Source: CAD feature listing. Evaluate the final solid. Frame: model axes, mm. Face numbers are marked on the shaded views. A direction names the side the tool comes from. Coordinates: 2 decimals unless noted, no trailing zeros. Write each loop counter-clockwise with the first axis right and the second up, starting at its lowest first coordinate (ties: lowest second). Pieces come first, ordered by that corner, then holes. Notation, with made-up numbers: M 87,-34.5 L 143,-34.5 A9 ccw 143,-23.5 Z; hole C -23,58 d3. An arc over 180 degrees is marked long. One line per item, written item: value. Start each with the question number.
Item 1: Pin query (flat end, axial travel): P1, Ø5, axis at x = 15, y = 13, coming from the -Z side; P2, Ø9.5, axis at x = 18.5, y = 10.5, coming from the +Z side; P3, Ø5, axis at y = 7, z = 20.5, coming from the -X side. Return the tip coordinate at first contact, or that it passes through.
Item 2: Ray query, L1, parallel to X at y = 10.25, z = 25.5; L2, parallel to Z at x = -1, y = 4; L3, parallel to Z at x = 43.5, y = 6. Return the intervals inside material, ascending. Write a range as from..to.
Item 3: Cut plane D-D, the plane z = 10. Output: boundary loops of the cut face in (x, y), then the cut area to 3 significant figures.
Item 4: Set-up query: the marked faces 1, 2, 3 and 4. Return all of +Z, -Z, +X, -X, +Y, -Y with unobstructed straight access to the full face (end or side cutting, diameter ignored); none if empty.
Item 5: Mould query, pull axis X, two halves, no side actions, for the marked faces 5, 6 and 7. Classes: released by +X, released by -X, zero draft, split by the parting line, or undercut.
Item 6: Cut plane A-A, the plane z = 18. Output: boundary loops of the cut face in (x, y), then the cut area to 3 significant figures.
Item 7: Cut plane C-C, the plane x = 26.5. Output: boundary loops of the cut face in (y, z), then the cut area to 3 significant figures.
Item 8: Cut plane B-B, the plane y = 8.75. Output: boundary loops of the cut face in (x, z).
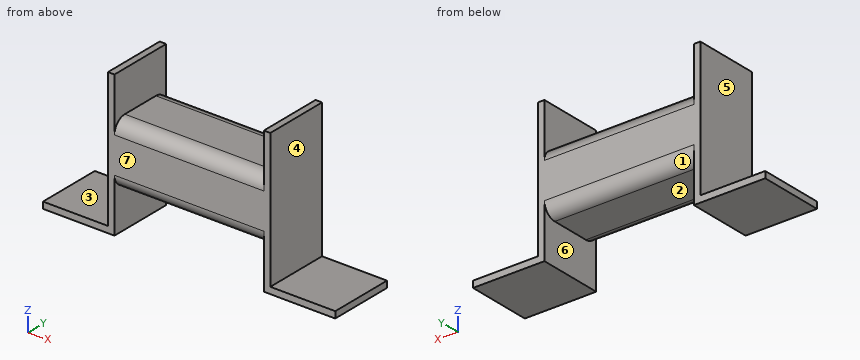
Autodesk Fusion 360 part; units mm, degrees
sketch "Sketch1" plane through (0, 0, 0) normal (0, 1, 0) x (1, 0, 0)
  line L0 (50, 0) -> (50, -15)
  line L1 (0, -15) -> (0, 0)
  line L2 (50, -15) -> (50, -27.5)
  line L3 (50, -27.5) -> (70, -27.5)
  line L4 (70, -27.5) -> (70, -29.5)
  line L5 (70, -29.5) -> (50, -29.5)
  line L6 (50, -29.5) -> (48, -29.5)
  line L7 (48, -29.5) -> (48, -17)
  line L8 (48, -17) -> (2, -17)
  line L9 (2, -17) -> (2, -29.5)
  line L10 (2, -29.5) -> (-20, -29.5)
  line L11 (-20, 14.5) -> (2, 14.5)
  line L12 (2, 14.5) -> (2, 2)
  line L13 (2, 2) -> (48, 2)
  line L14 (48, 2) -> (48, 14.5)
  line L15 (48, 14.5) -> (70, 14.5)
  line L16 (70, 14.5) -> (70, 12.5)
  line L17 (70, 12.5) -> (50, 12.5)
  line L18 (50, 12.5) -> (50, 0)
  line L19 (-20, 14.5) -> (-20, 12.5)
  line L20 (-20, 12.5) -> (0, 12.5)
  line L21 (0, 12.5) -> (0, 0)
  line L22 (-20, -29.5) -> (-20, -27.5)
  line L23 (-20, -27.5) -> (0, -27.5)
  line L24 (0, -27.5) -> (0, -15)
  dimension "d1" = 50
  dimension "d2" = 15
  dimension "d3" = 12.5
  dimension "d4" = 20
  dimension "d5" = 2
  dimension "d6" = 20
  dimension "d7" = 2
  dimension "d8" = 12.5
  dimension "d9" = 46
  dimension "d10" = 12.5
  dimension "d11" = 22
  dimension "d12" = 44
  dimension "d13" = 22
  dimension "d14" = 12.5
  dimension "d15" = 46
  dimension "d16" = 12.5
  dimension "d17" = 22
  dimension "d18" = 2
  dimension "d19" = 20
  dimension "d20" = 2
  dimension "d21" = 20
  dimension "d23" = 2
extrude "Extrude1" add sketch "Sketch1" along normal blind 20
fillet "Fillet1" radius 4 1 edges at (25, 20, 17)
fillet "Fillet2" radius 4 1 edges at (25, 0, 17)
fillet "Fillet3" radius 4 1 edges at (25, 20, -2)
fillet "Fillet4" radius 4 1 edges at (25, 0, -2)
sketch "Sketch2" plane through (50, 0, 0) normal (1, 0, 0) x (0, 0, -1)
  line L0 (-27.5, 0) -> (12.5, 0)
  line L1 (12.5, 0) -> (12.5, 20)
  line L2 (12.5, 20) -> (-27.5, 20)
  line L3 (-27.5, 20) -> (-27.5, 0)
extrude "Extrude2" cut 1 faces at (70, 6.6667, 28.1667) along direction (-1, 0, 0) blind 20
extrude "Extrude3" cut 1 faces at (-20, 6.6667, 28.8333) along direction (1, 0, 0) blind 20
From the geometry:
1. P1: stops at z = -2
1. P2: stops at z = 17
1. P3: stops at x = 0
2. L1: x = 0..2, 48..50
2. L2: z = -14.5..-12.5
2. L3: z = -2..17
3. outline: M 0,0 L 50,0 L 50,20 L 0,20 Z
3. area: 1,000 mm²
4. face 1: -Z, +Y
4. face 2: -Z, +Y, -Y
4. face 3: +Z, -X, +Y, -Y
4. face 4: +Z, +X, +Y, -Y
5. face 5: released by -X
5. face 6: undercut
5. face 7: zero draft
6. outline: M 0,0 L 2,0 L 2,20 L 0,20 Z; M 48,0 L 50,0 L 50,20 L 48,20 Z
6. area: 80.0 mm²
7. outline: M 0,2 A4 ccw 4,-2 L 16,-2 A4 ccw 20,2 L 20,13 A4 ccw 16,17 L 4,17 A4 ccw 0,13 Z
7. area: 366 mm²
8. outline: M -20,-14.5 L 2,-14.5 L 2,-2 L 48,-2 L 48,-14.5 L 70,-14.5 L 70,-12.5 L 50,-12.5 L 50,29.5 L 48,29.5 L 48,17 L 2,17 L 2,29.5 L 0,29.5 L 0,-12.5 L -20,-12.5 Z
